Geometry check sheet. Reference: the model listing, model coordinates, mm. A direction names the side the tool comes from. Give positions to 0.01 mm unless a question says otherwise; leave off trailing zeros. Write each loop counter-clockwise with the first axis right and the second up, starting at its lowest first coordinate (ties: lowest second). Pieces come first, ordered by that corner, then holes. Notation, with made-up numbers: (10, -26) - (39, -26) arc R15 ccw to (39, -1) - close; hole circle Ø3 at (48.25, 31.5). An arc over 180 degrees is marked (long way). Write item = value, one per line. Start each with the question number.
(1) Section check B-B, the plane z = 91. Enter the section's corners in (x, y), plus the area to 3 significant figures.
(2) Access from +Z, -Z, +X, -X, +Y, -Y to the whole of each face (thin tool, end or side, straight path). Record for faces 1 (the flat face through (-4, 425.45, 46)), 2 (the flat face through (-4, 431.8, 48)).
(3) Depth check by flat-ended pin: pin 1 Ø3 at (y, z) = (114, 11) entering from +X; pin 2 Ø2 at (y, z) = (-314, 110.5) entering from +X; pin 3 Ø6 at (x, y) = (6, 67) entering from +Z. Enter the tip coordinate at first touch or a pass-through.
(4) Section check A-A, the plane y = -194.5. Enter the section's corners in (x, z), plus the area to 3 significant figures.
(5) Section check D-D, the plane x = 153.5. Enter the section's corners in (y, z).
(6) Thickness scan on L1, parallel to Y at x = -56, z = 71.5; L2, parallel to X at y = 375.5, z = 63.5; L3, parallel to X at y = -151.5, z = 73.5. Record the ranges inside material, lowest first.
(7) Draft check along X on faces 3 (the flat face through (-135.22, -6.05, 62.61)), 4 (the flat face through (124.202, -5.956, 60.823)), 5 (the flat face through (131.48, -6.05, 64.39)), 6 (the flat face through (-127.729, -5.956, 59.144)). Enter one of: pulls with the +X half, pulls with the -X half, needs draft (parallel to the pull), parting line crosses it, or undercut.
(8) Section check C-C, the plane x = -36. Enter the section's corners in (y, z), plus the area to 3 significant figures.
```python
from build123d import *

# Parameters (mm, degrees)
F0_W     = 533.4
F0_H     = 863.6
F1_DEPTH = 127
F3_DEPTH = 2540
F4_T     = -6.35
F5_R     = 5.08
F6_DEPTH = 25.4


with BuildPart() as f1:
    # F0 (on Top) → F1 (new body)
    with BuildSketch(Plane.XY):
        Rectangle(F0_W, F0_H)
    extrude(amount=F1_DEPTH)

    # F2 (on face) → F3 (cut)
    with BuildSketch(Plane.XZ.offset(431.8)):
        Polygon((-266.7, 0), (0, 127), (-266.7, 127), align=None)
        Polygon((266.7, 127), (0, 127), (266.7, 0), align=None)
    extrude(amount=-F3_DEPTH, mode=Mode.SUBTRACT)

    # F4
    f4_openings = [f1.faces().sort_by_distance(p)[0] for p in [
        (0, 0, 0),
    ]]
    offset(amount=F4_T, openings=f4_openings)

    # F5 (on face) → F6 (join)
    with BuildSketch(Plane(origin=(0, 0, 0), x_dir=(1, 0, 0), z_dir=(0, 0, -1))):
        with Locations((-259.08, 424.18)):
            Circle(F5_R)
        with Locations((259.08, 424.18)):
            Circle(F5_R)
        with Locations((259.08, -424.18)):
            Circle(F5_R)
        with Locations((-259.08, -424.18)):
            Circle(F5_R)
    extrude(amount=F6_DEPTH)


solid = f1.part
```
Model answer:
q1.outline = (-75.6, -431.8) - (75.6, -431.8) - (75.6, 431.8) - (-75.6, 431.8) - close; hole (-60.83, -425.45) - (60.83, -425.45) - (60.83, 425.45) - (-60.83, 425.45) - close
q1.area = 27,100 mm²
q2.face_1 = -Z
q2.face_2 = +Z, -Z, +X, -X, +Y
q3.pin_1 = 246.75
q3.pin_2 = 36.75
q3.pin_3 = 125.57
q4.outline = (-266.7, 0) - (-251.93, 0) - (0, 119.97) - (251.93, 0) - (266.7, 0) - (0, 127) - close
q4.area = 3,650 mm²
q5.outline = (-431.8, 0) - (-425.45, 0) - (-425.45, 46.87) - (425.45, 46.87) - (425.45, 0) - (431.8, 0) - (431.8, 53.9) - (-431.8, 53.9) - close
q6.L1 = -431.8 to -425.45, 425.45 to 431.8
q6.L2 = -133.35 to -118.58, 118.58 to 133.35
q6.L3 = -112.35 to -97.58, 97.58 to 112.35
q7.face_3 = pulls with the -X half
q7.face_4 = undercut
q7.face_5 = pulls with the +X half
q7.face_6 = undercut
q8.outline = (-431.8, 0) - (-425.45, 0) - (-425.45, 102.82) - (425.45, 102.82) - (425.45, 0) - (431.8, 0) - (431.8, 109.86) - (-431.8, 109.86) - close
q8.area = 7,380 mm²
